```python
from build123d import *

# Parameters (mm, degrees)
F0_R     = 12.7
F1_DEPTH = 30.1625
F2_R     = 6.35
F3_DEPTH = 34.799
F2_W     = 54.5219902415
F2_H     = 22.3266
F4_DEPTH = 63.5
F5_DEPTH = 30.1625
F6_R     = 7.874
F7_DEPTH = 30.48
F8_DEPTH = 13.462
F9_DEPTH = 25.4
F10_R    = 7.874


with BuildPart() as f1:
    # F0 (on Front) → F1 (new body, symmetric)
    with BuildSketch(Plane.XZ):
        Polygon((85.852, 0), (22.352, 0), (22.352, -22.352), (91.8464, -22.352), align=None)
        with BuildLine():
            Line((22.352, -22.352), (22.352, 0))
            ThreePointArc((22.352, 0), (-15.8052507731, 15.8052507731), (0, -22.352))
            Line((0, -22.352), (22.352, -22.352))
        make_face()
        Circle(F0_R, mode=Mode.SUBTRACT)
    extrude(amount=F1_DEPTH, both=True)

    # F2 (on face) → F4 (cut, symmetric)
    with BuildSketch(Plane.XY):
        with Locations((-4.9089951208, 0)):
            Rectangle(F2_W, F2_H)
    extrude(amount=F4_DEPTH, both=True, mode=Mode.SUBTRACT)

    # F6
    f6_edges = [f1.edges().sort_by_distance(p)[0] for p in [
        (22.352, -20.6629, 0),
        (22.352, 20.6629, 0),
    ]]
    fillet(f6_edges, radius=F6_R)



with BuildPart() as f1b:
    # F0 (on Front) → F1, piece 2 (new body, symmetric)
    with BuildSketch(Plane.XZ):
        Polygon((117.2485877871, 0), (117.2485877871, -22.352), (194.2084, -22.352), (194.2084, 0), (150.0886, 0), align=None)
        with BuildLine():
            ThreePointArc((131.0386, 34.798), (127.4654323074, 16.0825969798), (117.2485877871, 0))
            Line((117.2485877871, 0), (150.0886, 0))
            Line((150.0886, 0), (150.0886, 34.798))
            Line((150.0886, 34.798), (131.0386, 34.798))
        make_face()
    extrude(amount=F1_DEPTH, both=True)

    # F2 (on face) → F3 (cut, through all)
    with BuildSketch(Plane.XY):
        with Locations((155.3464, 7.8105)):
            Circle(F2_R)
    extrude(amount=F3_DEPTH, mode=Mode.SUBTRACT)

    # F0 (on Front) → F5 (join, symmetric)
    with BuildSketch(Plane.XZ):
        with BuildLine():
            ThreePointArc((131.0386, 34.798), (127.4654323074, 16.0825969798), (117.2485877871, 0))
            Line((117.2485877871, 0), (150.0886, 0))
            Line((150.0886, 0), (150.0886, 34.798))
            Line((150.0886, 34.798), (131.0386, 34.798))
        make_face()
    extrude(amount=F5_DEPTH, both=True)


with BuildPart() as f7:
    # F0 (on Front) → F7 (new body)
    with BuildSketch(Plane.XZ):
        Polygon((108.2802, 0), (85.852, 0), (91.8464, -22.352), (117.2485877871, -22.352), (117.2485877871, 0), (117.2464, 0), align=None)
    extrude(amount=-F7_DEPTH)


with BuildPart() as f1_1:
    add(f1.part)

    add(f1b.part)  # F8 merges F1b

    add(f7.part)  # F8 merges F7
    # F0 (on Front) → F8 (join)
    with BuildSketch(Plane.XZ):
        Polygon((108.2802, 0), (85.852, 0), (91.8464, -22.352), (117.2485877871, -22.352), (117.2485877871, 0), (117.2464, 0), align=None)
    extrude(amount=F8_DEPTH)

    # F2 (on face) → F9 (cut)
    with BuildSketch(Plane.XY):
        with BuildLine():
            ThreePointArc((150.0886, 4.2498765771), (157.2085855439, 1.7396874514), (161.6964, 7.8105))
            ThreePointArc((161.6964, 7.8105), (157.2085855439, 13.8813125486), (150.0886, 11.3711234229))
            Line((150.0886, 11.3711234229), (150.0886, 4.2498765771))
        make_face()
    extrude(amount=-F9_DEPTH, mode=Mode.SUBTRACT)

    # F10
    f10_edges = [f1_1.edges().sort_by_distance(p)[0] for p in [
        (194.2084, 0, 0),
    ]]
    fillet(f10_edges, radius=F10_R)


solid = f1_1.part
```
Verification items for the finished model (mm, model axes). A direction names the side the tool comes from. Coordinates: 2 decimals unless noted, no trailing zeros. Loops run counter-clockwise (first coordinate to the right, second up) from the corner with the lowest first, then second, coordinate; pieces in that order, holes last. Notation, with made-up numbers: (-16, -13) - (-9, -13) arc R24 cw to (-9, 2) - close; hole circle Ø4 at (21, 85.25). An arc over 180 degrees is marked (long way). Put each result on its own line as item: value.
Item 1: Section check D-D (x = 157). Enter the section's corners in (y, z).
Conclusion:
outline: (-30.16, -22.35) - (1.68, -22.35) - (1.68, 0) - (-30.16, 0) - close; (13.94, -22.35) - (30.16, -22.35) - (30.16, 0) - (13.94, 0) - close
Item 2: Section check B-B (x = -6). Enter the section's corners in (y, z), then the cut area to 3 significant figures.
Conclusion:
outline: (-30.16, -21.53) - (-11.16, -21.53) - (-11.16, -11.19) - (-30.16, -11.19) - close; (-30.16, 11.19) - (-11.16, 11.19) - (-11.16, 21.53) - (-30.16, 21.53) - close; (11.16, -21.53) - (30.16, -21.53) - (30.16, -11.19) - (11.16, -11.19) - close; (11.16, 11.19) - (30.16, 11.19) - (30.16, 21.53) - (11.16, 21.53) - close
area: 786 mm2
Item 3: Section check C-C (z = 2). Enter the section's corners in (x, y).
Conclusion:
outline: (-22.26, -30.16) - (-12.54, -30.16) - (-12.54, -11.16) - (-22.26, -11.16) - close; (-22.26, 11.16) - (-12.54, 11.16) - (-12.54, 30.16) - (-22.26, 30.16) - close; (12.54, -30.16) - (23.94, -30.16) - (23.94, -11.16) - (12.54, -11.16) - close; (12.54, 11.16) - (23.94, 11.16) - (23.94, 30.16) - (12.54, 30.16) - close; (119.03, -30.16) - (150.09, -30.16) - (150.09, 30.16) - (119.03, 30.16) - close
Item 4: Gauge pin test, flat ends, axial feed: pin 1 Ø8 at (y, z) = (16.5, 9.5) entering from +X; pin 2 Ø18 at (x, y) = (67.5, -10) entering from +Z; pin 3 Ø11 at (x, z) = (97.5, -16) entering from -Y. Record the tip position at first contact, or that the pin passes through.
Conclusion:
pin 1: stops at x = 150.09
pin 2: stops at z = 0
pin 3: stops at y = -13.46
Item 5: Set-up check for faces 1 (the face through (88.807, 30.319, -11.02)), 2 (the face through (127.564, -0.422, 16.332)), 3 (the face through (88.89, -21.93, -11.33)), 4 (the face through (147, 30.162, 0)): record each of +Z, -Z, +X, -X, +Y, -Y from which the full face is reachable in a straight line by a thin tool's end or side.
Conclusion:
face 1: -Z, -X, +Y
face 2: +Z, +Y, -Y
face 3: +Z, -Y
face 4: +Z, -Z, +X, +Y
Item 6: Section check A-A (y = 26). Enter the section's corners in (x, z).
Conclusion:
outline: (0, -22.35) - (194.21, -22.35) - (194.21, -7.87) arc R7.87 ccw to (186.33, 0) - (150.09, 0) - (150.09, 34.8) - (131.04, 34.8) arc R50.8 cw to (117.25, 0) - (29.18, 0) arc R7.87 cw to (21.58, 5.82) arc R22.35 ccw (long way) to start; hole circle Ø25.4 at (0, 0)
Item 7: Scan lines: line 1 along Z through (x, y) = (0, 20); line 2 along Y through (x, z) = (156, -1.5); line 3 along Y through (x, z) = (155.5, -12.5). Record each from-to range of solid material in increasing order.
Conclusion:
line 1: z = -22.35 to -12.7, 12.7 to 22.35
line 2: y = -30.16 to 1.49, 14.13 to 30.16
line 3: y = -30.16 to 1.46, 14.16 to 30.16
Item 8: Draft check along Y on faces 5 (the face through (9, 11.163, -10)), 6 (the face through (117.249, -22, -11)), 7 (the face through (34, -30.162, -5)). Enter one of: pulls with the +Y half, pulls with the -Y half, needs draft (parallel to the pull), parting line crosses it, or undercut.
Conclusion:
face 5: undercut
face 6: needs draft
face 7: pulls with the -Y half
